Could you check a few things on this model? Use its own coordinates, in mm. A direction names the side the tool comes from. Give positions to 0.01 mm unless a question says otherwise; leave off trailing zeros. Loops run counter-clockwise (first coordinate to the right, second up) from the corner with the lowest first, then second, coordinate; pieces in that order, holes last. Notation, with made-up numbers: (19.5, -19) - (34.5, -19) arc R17 ccw to (34.5, 4) - close; hole circle Ø2 at (-7, -36.5). An arc over 180 degrees is marked (long way). Answer in a Markdown table with one row per item. Add a question column.
```python
from build123d import *

# Parameters (mm, degrees)
SKETCH1_W               = 39.6
SKETCH1_H               = 14.5
BOSS_EXTRUDE1_DEPTH     = 25
SKETCH2_W               = 54
SKETCH2_H               = 15
BOSS_EXTRUDE2_DEPTH     = 17.3
CUT_EXTRUDE1_DEPTH      = 42.880783183
CUT_EXTRUDE1_DEPTH_BACK = 42.880783183
CHAMFER1_SIZE           = 0.5
CHAMFER2_SIZE           = 0.5
CHAMFER3_SIZE           = 0.5
CHAMFER4_SIZE           = 0.5
TAP1_D                  = 4.134
LPATTERN1_COUNT         = 2
LPATTERN1_PITCH         = 25
LPATTERN1_COUNT_DIR2    = 2
LPATTERN1_PITCH_DIR2    = 46


with BuildPart() as part:
    # Sketch1 → Boss-Extrude1 (new, symmetric)
    with BuildSketch(Plane(origin=(0, 0, 0), x_dir=(0, 0, -1), z_dir=(1, 0, 0))):
        with Locations((0, 12.25)):
            Rectangle(SKETCH1_W, SKETCH1_H)
    extrude(amount=BOSS_EXTRUDE1_DEPTH, both=True)

    # Sketch2 → Boss-Extrude2 (add, symmetric)
    with BuildSketch(Plane(origin=(0, 0, 0), x_dir=(0, 0, -1), z_dir=(1, 0, 0))):
        with Locations((0, 12.5)):
            Rectangle(SKETCH2_W, SKETCH2_H)
    extrude(amount=BOSS_EXTRUDE2_DEPTH, both=True)

    # Sketch3 → Cut-Extrude1 (cut, two sides: drawn at the far end of the back side and taken through both)
    with BuildSketch(Plane(origin=(0, 0, 0), x_dir=(0, 0, -1), z_dir=(1, 0, 0)).offset(-CUT_EXTRUDE1_DEPTH_BACK)):
        with BuildLine():
            Line((-9.7, 11), (9.7, 11))
            Line((9.7, 11), (10, 10.7))
            Line((10, 10.7), (10, 10.221039482))
            Line((10, 10.221039482), (9.455259378, 9.911421591))
            ThreePointArc((9.455259378, 9.911421591), (9.0228024, 9.564639684), (8.720500078, 9.1))
            Line((8.720500078, 9.1), (7.5, 9.1))
            Line((7.5, 9.1), (7.5, 7.9))
            Line((7.5, 7.9), (8.724976489, 7.9))
            ThreePointArc((8.724976489, 7.9), (9.018551739, 7.450071616), (9.434780564, 7.110401858))
            Line((9.434780564, 7.110401858), (10, 6.778960518))
            Line((10, 6.778960518), (10, 0))
            Line((10, 0), (-10, 0))
            Line((-10, 0), (-10, 6.778960518))
            Line((-10, 6.778960518), (-9.434780564, 7.110401858))
            ThreePointArc((-9.434780564, 7.110401858), (-9.018551739, 7.450071616), (-8.724976489, 7.9))
            Line((-8.724976489, 7.9), (-7.5, 7.9))
            Line((-7.5, 7.9), (-7.5, 9.1))
            Line((-7.5, 9.1), (-8.720500078, 9.1))
            ThreePointArc((-8.720500078, 9.1), (-9.0228024, 9.564639684), (-9.455259378, 9.911421591))
            Line((-9.455259378, 9.911421591), (-10, 10.221039482))
            Line((-10, 10.221039482), (-10, 10.7))
            Line((-10, 10.7), (-9.7, 11))
        make_face()
    extrude(amount=CUT_EXTRUDE1_DEPTH + CUT_EXTRUDE1_DEPTH_BACK, mode=Mode.SUBTRACT)

    # Chamfer1
    chamfer1_edges = [part.edges().sort_by_distance(p)[0] for p in [
        (-21.15, 19.5, 19.8),
        (-21.15, 19.5, -19.8),
        (21.15, 19.5, 19.8),
        (21.15, 19.5, -19.8),
    ]]
    chamfer(chamfer1_edges, length=CHAMFER1_SIZE)

    # Chamfer2
    chamfer2_edges = [part.edges().sort_by_distance(p)[0] for p in [
        (0, 20, 27),
        (0, 20, -27),
    ]]
    chamfer(chamfer2_edges, length=CHAMFER2_SIZE)

    # Chamfer3
    chamfer3_edges = [part.edges().sort_by_distance(p)[0] for p in [
        (-21.15, 5, -19.8),
        (-21.15, 5, 19.8),
        (21.15, 5, -19.8),
        (21.15, 5, 19.8),
    ]]
    chamfer(chamfer3_edges, length=CHAMFER3_SIZE)

    # Chamfer4
    chamfer4_edges = [part.edges().sort_by_distance(p)[0] for p in [
        (0, 5, 27),
        (0, 5, -27),
    ]]
    chamfer(chamfer4_edges, length=CHAMFER4_SIZE)

    # Tap1 (through all)
    with Locations(Plane(origin=(0, 20, 0), x_dir=(1, 0, 0), z_dir=(0, 1, 0))):
        with Locations((-12.5, 23)):
            tap1 = Hole(TAP1_D / 2)

    # LPattern1: Tap1 2 × 2
    with Locations(*[(i * LPATTERN1_PITCH, 0, j * LPATTERN1_PITCH_DIR2) for i in range(LPATTERN1_COUNT) for j in range(LPATTERN1_COUNT_DIR2) if (i, j) != (0, 0)]):
        add(tap1, mode=Mode.SUBTRACT)


solid = part.part
```
(1) On a 3-axis mill with a long thin cutter (end or side, diameter ignored), from which of +Z, -Z, +X, -X, +Y, -Y can I reach the whole of each face in a straight line? I mean faces 4 (the flat face through (0, 9.1, -8)), 5 (the flat face through (0, 7.9, 8)), 6 (the flat face through (21, 12, 19.8)). Say none if no direction works.
(2) Please list where these lines run through material, in increasing order: line 1 (Z direction, x = -12.5, y = 17); line 2 (X direction, y = 15.75, z = 23); line 3 (Z direction, x = -0.5, y = 6.5).
(3) I want a section at D-D on x = -12.5. State how many separate pieces and enclosed holes the cut face has, then the cut area to 3 significant figures.
(4) I want a section at B-B on y = 17.25. Please give me the cut outline in (x, z), then the cut area to 3 significant figures.
(5) I want a section at A-A on z = 23. Please give me the cut outline in (x, y).
(6) We'd pull the mould along X, two halves only. Please class faces 1 (the flat face through (25, 14, 0)), 2 (the cylindrical face through (-10.98, 12.39, 21.6)), 3 (the flat face through (0, 11, 0)): pulls with the +X half, pulls with the -X half, needs draft (parallel to the pull), parting line crosses it, or undercut.
(7) For pin 1 Ø3.5 at (x, z) = (-12.5, 23) entering from +Y; pin 2 Ø10 at (x, z) = (5.5, 0.5) entering from -Y; pin 3 Ø6 at (x, y) = (-22, 9.5) entering from +Z; pin 4 Ø1.3 at (x, z) = (3.5, -8) entering from -Y, each with a flat end and sliding along its axis, tell me the tip position at first contact or that it passes through.
Reported:
| question | item | result |
|---|---|---|
| 1 | face 4 | +X, -X |
| 1 | face 5 | +X, -X, -Y |
| 1 | face 6 | +Z, +X, +Y, -Y |
| 2 | line 1 | -27 to -25.07, -20.93 to 20.93, 25.07 to 27 |
| 2 | line 2 | -17.3 to -14.57, -10.43 to 10.43, 14.57 to 17.3 |
| 2 | line 3 | -27 to -10, 10 to 27 |
| 3 | separate pieces | 3 |
| 3 | enclosed holes | 0 |
| 3 | area | 575 mm² |
| 4 | outline | (-25, -19.8) - (-17.3, -19.8) - (-17.3, -27) - (17.3, -27) - (17.3, -19.8) - (25, -19.8) - (25, 19.8) - (17.3, 19.8) - (17.3, 27) - (-17.3, 27) - (-17.3, 19.8) - (-25, 19.8) - close; hole circle Ø4.13 at (-12.5, -23); hole circle Ø4.13 at (-12.5, 23); hole circle Ø4.13 at (12.5, -23); hole circle Ø4.13 at (12.5, 23) |
| 4 | area | 2,420 mm² |
| 5 | outline | (-17.3, 5) - (-14.57, 5) - (-14.57, 20) - (-17.3, 20) - close; (-10.43, 5) - (10.43, 5) - (10.43, 20) - (-10.43, 20) - close; (14.57, 5) - (17.3, 5) - (17.3, 20) - (14.57, 20) - close |
| 6 | face 1 | pulls with the +X half |
| 6 | face 2 | undercut |
| 6 | face 3 | needs draft |
| 7 | pin 1 | through |
| 7 | pin 2 | y = 11 |
| 7 | pin 3 | z = 19.8 |
| 7 | pin 4 | y = 7.9 |
